```python
from build123d import *

# Parameters (mm, degrees)
SKETCH1_R           = 9
SKETCH1_R_2         = 3
SKETCH1_R_3         = 1.65
BOSS_EXTRUDE1_DEPTH = 6.35
CUT_EXTRUDE1_DEPTH  = 10
FILLET1_R           = 2


with BuildPart() as part:
    # Sketch1 → Boss-Extrude1 (new body)
    with BuildSketch(Plane.XY):
        with BuildLine():
            Line((-15, 15), (-15, -15))
            ThreePointArc((-15, -15), (-14.275727836, -25.159324804), (-12.117561222, -35.113156605))
            ThreePointArc((-12.117561222, -35.113156605), (-11.640196728, -62.923473964), (-25.409366876, -87.090633124))
            ThreePointArc((-25.409366876, -87.090633124), (-27.067678424, -89.572471742), (-27.65, -92.5))
            Line((-27.65, -92.5), (-27.65, -97))
            ThreePointArc((-27.65, -97), (-26.771320344, -99.121320344), (-24.65, -100))
            Line((-24.65, -100), (24.65, -100))
            ThreePointArc((24.65, -100), (26.771320344, -99.121320344), (27.65, -97))
            Line((27.65, -97), (27.65, -92.5))
            ThreePointArc((27.65, -92.5), (27.067678424, -89.572471742), (25.409366876, -87.090633124))
            ThreePointArc((25.409366876, -87.090633124), (11.640196728, -62.923473964), (12.117561222, -35.113156605))
            ThreePointArc((12.117561222, -35.113156605), (14.275727836, -25.159324804), (15, -15))
            Line((15, -15), (15, 15))
            ThreePointArc((15, 15), (14.275727836, 25.159324804), (12.117561222, 35.113156605))
            ThreePointArc((12.117561222, 35.113156605), (11.640196728, 62.923473964), (25.409366876, 87.090633124))
            ThreePointArc((25.409366876, 87.090633124), (27.067678424, 89.572471742), (27.65, 92.5))
            Line((27.65, 92.5), (27.65, 97))
            ThreePointArc((27.65, 97), (26.771320344, 99.121320344), (24.65, 100))
            Line((24.65, 100), (-24.65, 100))
            ThreePointArc((-24.65, 100), (-26.771320344, 99.121320344), (-27.65, 97))
            Line((-27.65, 97), (-27.65, 92.5))
            ThreePointArc((-27.65, 92.5), (-27.067678424, 89.572471742), (-25.409366876, 87.090633124))
            ThreePointArc((-25.409366876, 87.090633124), (-11.640196728, 62.923473964), (-12.117561222, 35.113156605))
            ThreePointArc((-12.117561222, 35.113156605), (-14.275727836, 25.159324804), (-15, 15))
        make_face()
        Circle(SKETCH1_R, mode=Mode.SUBTRACT)
        with Locations((0, 44.9961)):
            Circle(SKETCH1_R_2, mode=Mode.SUBTRACT)
        with Locations((20, 92.5)):
            Circle(SKETCH1_R_3, mode=Mode.SUBTRACT)
        with Locations((-20, 92.5)):
            Circle(SKETCH1_R_3, mode=Mode.SUBTRACT)
        with Locations((-20, -92.5)):
            Circle(SKETCH1_R_3, mode=Mode.SUBTRACT)
        with Locations((20, -92.5)):
            Circle(SKETCH1_R_3, mode=Mode.SUBTRACT)
        with BuildLine():
            Line((3, -43.0351625), (3, -46.9570375))
            ThreePointArc((3, -46.9570375), (0, -49.9570375), (-3, -46.9570375))
            Line((-3, -46.9570375), (-3, -43.0351625))
            ThreePointArc((-3, -43.0351625), (0, -40.0351625), (3, -43.0351625))
        make_face(mode=Mode.SUBTRACT)
    extrude(amount=BOSS_EXTRUDE1_DEPTH)

    # Sketch3 → Cut-Extrude1 (cut)
    with BuildSketch(Plane.XY.offset(6.35)):
        with BuildLine():
            Line((-8.5, 101), (-8.5, 86))
            ThreePointArc((-8.5, 86), (-7.914213562, 84.585786438), (-6.5, 84))
            Line((-6.5, 84), (6.5, 84))
            ThreePointArc((6.5, 84), (7.914213562, 84.585786438), (8.5, 86))
            Line((8.5, 86), (8.5, 101))
            Line((8.5, 101), (-8.5, 101))
        make_face()
    extrude(amount=-CUT_EXTRUDE1_DEPTH, mode=Mode.SUBTRACT)

    # Fillet1
    fillet1_edges = [part.edges().sort_by_distance(p)[0] for p in [
        (-8.5, 100, 3.175),
        (8.5, 100, 3.175),
    ]]
    fillet(fillet1_edges, radius=FILLET1_R)


solid = part.part
```
Geometry: final body of the model. Coordinates: model frame, mm. A direction names the side the tool comes from. Round coordinates to 2 decimals unless told otherwise and drop trailing zeros. Loops run counter-clockwise (first coordinate to the right, second up) from the corner with the lowest first, then second, coordinate; pieces in that order, holes last. Notation, with made-up numbers: (-22, 60.25) -> (-15, 60.25) arc R25 ccw to (-15, 76.25) -> close; hole circle Ø8 at (-6, -4). An arc over 180 degrees is marked (long way). Use one line per item in the form item = value. Start each with the question number.
1) Access query for faces 1 (the cylindrical face through (19.6, 90.9, 3.1)), 2 (the cylindrical face through (27.084, -89.611, 3.131)), 3 (the cylindrical face through (-27.05, -89.53, 3.13)). Directions: +Z, -Z, +X, -X, +Y, -Y. A direction counts if a zero-diameter tool reaches every point of the face in a straight line with its end or side. Return the directions, or none.
2) Section D-D on y = -67.5. Output: boundary loops of the cut face in (x, z).
3) Line query: L1, parallel to Y at x = 0, z = 4.5; L2, parallel to X at y = 92.5, z = 3; L3, parallel to Y at x = -19, z = 6. Output: solid intervals per line, ascending.
4) Section A-A on x = 0. Output: boundary loops of the cut face in (y, z).
5) Draft query along X for faces 4 (the flat face through (12, 1, 6.35)), 5 (the cylindrical face through (0.066, -49.956, 3.131)), 6 (the cylindrical face through (14.3, 25, 3.1)), 7 (the cylindrical face through (-0.39, 47.97, 3.13)). Return one class per face: released by +X, released by -X, zero draft, split by the parting line, or undercut.
6) First-contact query: P1, Ø3, axis at x = 13.5, y = 43, coming from the -Z side; P2, Ø1, axis at y = -9.5, z = 2, coming from the +X side; P3, Ø3, axis at y = -44.5, z = 4.5, coming from the -X side; P4, Ø10, axis at x = -2, y = -39, coming from the -Z side. Flat tips, straight axial feed; report the tip coordinate or a pass-through.
7) Section B-B on z = 2. Give the number of separate pieces and of enclosed holes in the cut face, then the cut area to 3 significant figures.
8) Section C-C on y = -37. Output: boundary loops of the cut face in (x, z).
Response:
q1.face_1 = +Z, -Z
q1.face_2 = +Z, -Z, +X
q1.face_3 = +Z, -Z, -X
q2.outline = (-13.04, 0) -> (13.04, 0) -> (13.04, 6.35) -> (-13.04, 6.35) -> close
q3.L1 = -100 to -49.96, -40.04 to -9, 9 to 42, 48 to 84
q3.L2 = -27.65 to -21.65, -18.35 to -8.5, 8.5 to 18.35, 21.65 to 27.65
q3.L3 = -100 to -93.81, -91.19 to -79.32, 79.32 to 91.19, 93.81 to 100
q4.outline = (-100, 0) -> (-49.96, 0) -> (-49.96, 6.35) -> (-100, 6.35) -> close; (-40.04, 0) -> (-9, 0) -> (-9, 6.35) -> (-40.04, 6.35) -> close; (9, 0) -> (42, 0) -> (42, 6.35) -> (9, 6.35) -> close; (48, 0) -> (84, 0) -> (84, 6.35) -> (48, 6.35) -> close
q5.face_4 = zero draft
q5.face_5 = undercut
q5.face_6 = released by +X
q5.face_7 = undercut
q6.P1 = through
q6.P2 = 15
q6.P3 = -10.45
q6.P4 = 0
q7.separate_pieces = 1
q7.enclosed_holes = 7
q7.area = 5,630 mm^2
q8.outline = (-11.6, 0) -> (11.6, 0) -> (11.6, 6.35) -> (-11.6, 6.35) -> close
